Input: part model. Units: mm. Frame: model coordinates. A direction names the side the tool comes from. Coordinates: 2 decimals unless noted, no trailing zeros. Order: outer loops, then holes, each group sorted by start corner. A loop starts at its lowest first (then second) coordinate and runs counter-clockwise, first axis right, second up. Notation, with made-up numbers: (60, 76) - (95, 76) arc R29 ccw to (95, 100) - close; hole circle Ø5 at (-36.75, -21.5). An arc over 180 degrees is marked (long way). Answer as CSV lines item,"result". Start each with the question number.
Item 1: First-contact query: pin 1 (10 mm diameter, centred on y = -9.5, z = 17.5, fed in from -X); pin 2 (8 mm diameter, centred on x = -12, y = 4, fed in from +Z); pin 3 (10 mm diameter, centred on x = -1, y = -10.5, fed in from +Z). Flat tips, straight axial feed; report the tip coordinate or a pass-through.
Item 2: Section D-D (y = 0). Output: boundary loops of the cut face in (x, z), and give its area (3 significant figures).
Item 3: Access query for faces 5 (the flat face through (10, 0, 3)), 6 (the flat face through (0, -7.5, 33)), 7 (the flat face through (-2, 5, 32)). Directions: +Z, -Z, +X, -X, +Y, -Y. A direction counts if a zero-diameter tool reaches every point of the face in a straight line with its end or side. Return the directions, or none.
Item 4: Draft query along X for faces 1 (the cylindrical face through (9.659, -11.538, 1.521)), 2 (the flat face through (-15, 0, 1)), 3 (the flat face through (0.1, -14.7, 5.8)), 4 (the cylindrical face through (-10.341, 8.462, 1.521)). Return one class per face: +X half, -X half, draft (parallel to the pull), parting line (faces both ways), or undercut.
Item 5: Section A-A (z = 43). Output: boundary loops of the cut face in (x, y).
Item 6: Section C-C (x = -10). Output: boundary loops of the cut face in (y, z) (3 decimals), and give its area (3 significant figures).
Item 7: Section B-B (y = 6). Output: boundary loops of the cut face in (x, z).
Item 8: Material intervals for line 1 along Y through (x, z) = (10, 1.7) (3 decimals); line 2 along X through (y, z) = (-4, 45.5); line 3 along Z through (x, y) = (14, -6), sorted ascending.
from build123d import *

# Parameters (mm, degrees)
SKETCH1_W           = 30
SKETCH1_H           = 35
BOSS_EXTRUDE1_DEPTH = 3
SKETCH2_W           = 4
SKETCH2_H           = 35
BOSS_EXTRUDE2_DEPTH = 55
FILLET1_R           = 10
FILLET2_R           = 10
SKETCH3_R           = 1.575
CUT_EXTRUDE1_DEPTH  = 55
SKETCH4_R           = 1.25
CUT_EXTRUDE2_DEPTH  = 55
SKETCH5_W           = 53.614570856
SKETCH5_H           = 10
CUT_EXTRUDE3_DEPTH  = 55
FILLET3_R           = 10
CUT_EXTRUDE4_DEPTH  = 55
FILLET4_R           = 10
FILLET5_R           = 3


with BuildPart() as part:
    # Sketch1 → Boss-Extrude1 (new body)
    with BuildSketch(Plane.XY):
        Rectangle(SKETCH1_W, SKETCH1_H)
    extrude(amount=BOSS_EXTRUDE1_DEPTH)

    # Sketch2 → Boss-Extrude2 (add)
    with BuildSketch(Plane.XY.offset(3)):
        Rectangle(SKETCH2_W, SKETCH2_H)
    extrude(amount=BOSS_EXTRUDE2_DEPTH)

    # Fillet1
    fillet1_edges = [part.edges().sort_by_distance(p)[0] for p in [
        (0, 17.5, 58),
        (0, -17.5, 58),
    ]]
    fillet(fillet1_edges, radius=FILLET1_R)

    # Fillet2
    fillet2_edges = [part.edges().sort_by_distance(p)[0] for p in [
        (15, -17.5, 1.5),
        (-15, -17.5, 1.5),
        (-15, 17.5, 1.5),
        (15, 17.5, 1.5),
    ]]
    fillet(fillet2_edges, radius=FILLET2_R)

    # Sketch3 → Cut-Extrude1 (cut)
    with BuildSketch(Plane.XY.offset(3)):
        with Locations((-10, 10)):
            Circle(SKETCH3_R)
        with Locations((10, -10)):
            Circle(SKETCH3_R)
        with Locations((10, 10)):
            Circle(SKETCH3_R)
        with Locations((-10, -10)):
            Circle(SKETCH3_R)
    extrude(amount=-CUT_EXTRUDE1_DEPTH, mode=Mode.SUBTRACT)

    # Sketch4 → Cut-Extrude2 (cut)
    with BuildSketch(Plane(origin=(2, 0, 0), x_dir=(0, 0, -1), z_dir=(1, 0, 0))):
        with Locations((-43, 0)):
            Circle(SKETCH4_R)
    extrude(amount=-CUT_EXTRUDE2_DEPTH, mode=Mode.SUBTRACT)

    # Sketch5 → Cut-Extrude3 (cut)
    with BuildSketch(Plane(origin=(2, 0, 0), x_dir=(0, 0, -1), z_dir=(1, 0, 0))):
        with Locations((-39.807285428, -12.5)):
            Rectangle(SKETCH5_W, SKETCH5_H)
    extrude(amount=-CUT_EXTRUDE3_DEPTH, mode=Mode.SUBTRACT)

    # Fillet3
    fillet3_edges = [part.edges().sort_by_distance(p)[0] for p in [
        (0, -7.5, 58),
    ]]
    fillet(fillet3_edges, radius=FILLET3_R)

    # Sketch6 → Cut-Extrude4 (cut)
    with BuildSketch(Plane(origin=(2, 0, 0), x_dir=(0, 0, -1), z_dir=(1, 0, 0))):
        Polygon((-13, -7.5), (-3, -17.5), (-13, -17.5), align=None)
    extrude(amount=-CUT_EXTRUDE4_DEPTH, mode=Mode.SUBTRACT)

    # Fillet4
    fillet4_edges = [part.edges().sort_by_distance(p)[0] for p in [
        (0, -7.5, 13),
    ]]
    fillet(fillet4_edges, radius=FILLET4_R)

    # Fillet5
    fillet5_edges = [part.edges().sort_by_distance(p)[0] for p in [
        (2, 0, 3),
        (-2, 0, 3),
    ]]
    fillet(fillet5_edges, radius=FILLET5_R - 0.0001)  # a hair under: the kernel refuses the full size


solid = part.part
Determined:
1,pin 1,"stops at x = -2"
1,pin 2,"stops at z = 3"
1,pin 3,"stops at z = 54"
2,outline,"(-15, 0) - (15, 0) - (15, 3) - (5, 3) arc R3 cw to (2, 6) - (2, 41.75) - (-2, 41.75) - (-2, 6) arc R3 cw to (-5, 3) - (-15, 3) - close; (-2, 44.25) - (2, 44.25) - (2, 57.68) - (-2, 57.68) - close"
2,area,"303 mm^2"
3,face 5,"+Z, +X, +Y, -Y"
3,face 6,"+Z, +X, -X, -Y"
3,face 7,"+Z, -X, +Y, -Y"
4,face 1,"undercut"
4,face 2,"-X half"
4,face 3,"draft"
4,face 4,"undercut"
5,outline,"(-2, -7.5) - (2, -7.5) - (2, -1.25) - (-2, -1.25) - close; (-2, 1.25) - (2, 1.25) - (2, 17.5) - (-2, 17.5) - close"
6,outline,"(-16.16, 0) - (-11.575, 0) - (-11.575, 3) - (-16.16, 3) - close; (-8.425, 0) - (8.425, 0) - (8.425, 3) - (-8.425, 3) - close; (11.575, 0) - (16.16, 0) - (16.16, 3) - (11.575, 3) - close"
6,area,"78.1 mm^2"
7,outline,"(-15, 0) - (15, 0) - (15, 3) - (5, 3) arc R3 cw to (2, 6) - (2, 58) - (-2, 58) - (-2, 6) arc R3 cw to (-5, 3) - (-15, 3) - close"
8,line 1,"y = -16.16 to -11.575, -8.425 to 8.425, 11.575 to 16.16"
8,line 2,"x = -2 to 2"
8,line 3,"z = 0 to 3"
